from build123d import *

# Parameters (mm, degrees)
SKETCH1_W           = 107.95
SKETCH1_H           = 44.45
BOSS_EXTRUDE1_DEPTH = 69.85
SKETCH2_W           = 18.973953495
SKETCH2_H           = 6.048241647
CUT_EXTRUDE1_DEPTH  = 141.986
SKETCH3_W           = 38.080163228
SKETCH3_H           = 3.050825249
SKETCH3_W_2         = 51.430009823
CUT_EXTRUDE3_DEPTH  = 141.986
CUT_EXTRUDE4_DEPTH  = 141.986
SKETCH8_R           = 114.3
CUT_EXTRUDE6_DEPTH  = 33.274
SKETCH12_R          = 119.126
CUT_EXTRUDE7_DEPTH  = 7.874
SKETCH13_R          = 6.35
CUT_EXTRUDE8_DEPTH  = 20.574
SKETCH14_R          = 76.2
CUT_EXTRUDE9_DEPTH  = 7.874
SKETCH15_R          = 6.35
CUT_EXTRUDE10_DEPTH = 20.574
SKETCH16_R          = 4.826
CUT_EXTRUDE11_DEPTH = 81.28


with BuildPart() as part:
    # Sketch1 → Boss-Extrude1 (new body)
    with BuildSketch(Plane(origin=(0, 0, 0), x_dir=(1, 0, 0), z_dir=(0, 1, 0))):
        with Locations((2.544990177, 0.698624754)):
            Rectangle(SKETCH1_W, SKETCH1_H)
    extrude(amount=BOSS_EXTRUDE1_DEPTH)

    # Sketch2 → Cut-Extrude1 (cut)
    with BuildSketch(Plane(origin=(56.519990177, 0, 0), x_dir=(0, 0, -1), z_dir=(1, 0, 0))):
        with Locations((0.660601501, 3.024120824)):
            Rectangle(SKETCH2_W, SKETCH2_H)
    extrude(amount=-CUT_EXTRUDE1_DEPTH, mode=Mode.SUBTRACT)

    # Sketch3 → Cut-Extrude3 (cut)
    with BuildSketch(Plane.XY.offset(21.526375246)):
        with Locations((37.479908563, 1.525412625)):
            Rectangle(SKETCH3_W, SKETCH3_H)
        with Locations((-25.715004912, 1.525412625)):
            Rectangle(SKETCH3_W_2, SKETCH3_H)
    extrude(amount=-CUT_EXTRUDE3_DEPTH, mode=Mode.SUBTRACT)

    # Sketch7 → Cut-Extrude4 (cut)
    with BuildSketch(Plane.XY.offset(21.526375246)):
        Polygon((-51.430009823, 54.102), (-42.337897784, 69.85), (-51.430009823, 69.85), align=None)
    extrude(amount=-CUT_EXTRUDE4_DEPTH, mode=Mode.SUBTRACT)

    # Sketch8 → Cut-Extrude6 (cut)
    with BuildSketch(Plane(origin=(0, 69.85, 0), x_dir=(1, 0, 0), z_dir=(0, 1, 0))):
        with Locations((112.145990177, 0.825624754)):
            Circle(SKETCH8_R)
    extrude(amount=-CUT_EXTRUDE6_DEPTH, mode=Mode.SUBTRACT)

    # Sketch12 → Cut-Extrude7 (cut)
    with BuildSketch(Plane(origin=(0, 36.576, 0), x_dir=(1, 0, 0), z_dir=(0, 1, 0))):
        with Locations((112.145990177, 0.825624754)):
            Circle(SKETCH12_R)
    extrude(amount=CUT_EXTRUDE7_DEPTH, mode=Mode.SUBTRACT)

    # Sketch13 → Cut-Extrude8 (cut)
    with BuildSketch(Plane(origin=(0, 36.576, 0), x_dir=(1, 0, 0), z_dir=(0, 1, 0))):
        with Locations(Location((37.469990177, 0.825624754, 0), (0, 0, 270))):
            Circle(SKETCH13_R)
    extrude(amount=-CUT_EXTRUDE8_DEPTH, mode=Mode.SUBTRACT)

    # Sketch14 → Cut-Extrude9 (cut)
    with BuildSketch(Plane(origin=(0, 36.576, 0), x_dir=(1, 0, 0), z_dir=(0, 1, 0))):
        with Locations((107.319990177, 0.825624754)):
            Circle(SKETCH14_R)
    extrude(amount=-CUT_EXTRUDE9_DEPTH, mode=Mode.SUBTRACT)

    # Sketch15 → Cut-Extrude10 (cut)
    with BuildSketch(Plane(origin=(0, 69.85, 0), x_dir=(1, 0, 0), z_dir=(0, 1, 0))):
        with Locations(Location((-26.030009823, 0.825624754, 0), (0, 0, 270))):
            Circle(SKETCH15_R)
    extrude(amount=-CUT_EXTRUDE10_DEPTH, mode=Mode.SUBTRACT)

    # Sketch16 → Cut-Extrude11 (cut)
    with BuildSketch(Plane(origin=(0, 69.85, 0), x_dir=(1, 0, 0), z_dir=(0, 1, 0))):
        with Locations(Location((-26.030009823, 0.825624754, 0), (0, 0, 270))):
            Circle(SKETCH16_R)
        with Locations(Location((37.469990177, 0.825624754, 0), (0, 0, 270))):
            Circle(SKETCH16_R)
    extrude(amount=-CUT_EXTRUDE11_DEPTH, mode=Mode.SUBTRACT)


solid = part.part
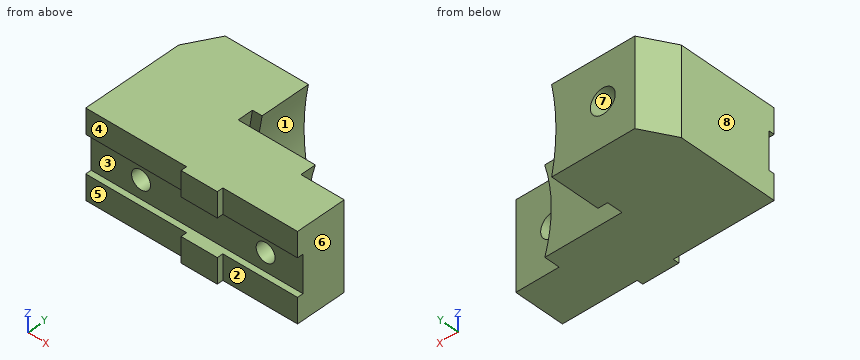
Geometry check sheet. Reference: the model listing, model coordinates, mm. Face numbers are marked on the shaded views. A direction names the side the tool comes from. Give positions to 0.01 mm unless a question says otherwise; leave off trailing zeros. Order: outer loops, then holes, each group sorted by start corner. A loop starts at its lowest first (then second) coordinate and runs counter-clockwise, first axis right, second up. Notation, with made-up numbers: M 11,37 L 35,37 A25 cw 35,61 Z; hole C 49.5,83.25 d1. An arc over 180 degrees is marked long. Use a Markdown table: item, result.
Item 1: Tool access check on the marked faces 1, 2, 3 and 4. Record the directions out of +Z, -Z, +X, -X, +Y, -Y that give a thin tool (end or side, any length) a straight path to the whole face; none if there is none.
Answers follow:
| item | result |
|---|---|
| face 1 | +X, +Y |
| face 2 | +Z, -Z, +X, -Y |
| face 3 | +X, -X, -Y |
| face 4 | +Z, -Z, -X, -Y |
Item 2: Section check B-B (z = -2). Record the cut outline in (x, y), and give its area (3 significant figures).
Answers follow:
| item | result |
|---|---|
| outline | M -51.43,6.05 L -30.71,6.05 L -30.71,49.28 L -32.27,49.28 L -32.27,69.85 L -42.34,69.85 L -51.43,54.1 Z; M -21.35,6.05 L 32.79,6.05 L 32.79,16 L 31.23,16 L 31.23,28.7 L 31.13,28.7 L 31.13,36.58 L -6.97,36.58 L -6.97,44.45 L -2.15,44.45 L -2.15,69.85 L -19.79,69.85 L -19.79,49.28 L -21.35,49.28 Z; M 42.15,6.05 L 56.52,6.05 L 56.52,28.7 L 43.71,28.7 L 43.71,16 L 42.15,16 Z |
| area | 3,710 mm2 |
Item 3: Material ranges on line 1 along X through (y, z) = (20.5, 1); line 2 along Y through (x, z) = (-5.5, 9.5); line 3 along Y through (x, z) = (13, 3), recorded low to high.
Answers follow:
| item | result |
|---|---|
| line 1 | x = -51.43 to -30.5, -21.56 to 31.39, 43.55 to 56.52 |
| line 2 | y = 3.05 to 36.58, 44.45 to 69.85 |
| line 3 | y = 6.05 to 36.58 |
Item 4: Depth check by flat-ended pin: P1, Ø1.5, axis at y = 1, z = 16.5, coming from the +X side; P2, Ø14, axis at x = -25.5, z = -14, coming from the -Y side; P3, Ø12.5, axis at x = 20, z = 6, coming from the +Y side. Enter the tip coordinate at first touch or a pass-through.
Answers follow:
| item | result |
|---|---|
| P1 | stops at x = 18.44 |
| P2 | stops at y = 3.05 |
| P3 | stops at y = 36.58 |
Item 5: Draft check along X on the marked faces 5, 6, 7 and 8. Enter one of: +X half, -X half, draft (parallel to the pull), parting line (faces both ways), or undercut.
Answers follow:
| item | result |
|---|---|
| face 5 | draft |
| face 6 | +X half |
| face 7 | undercut |
| face 8 | -X half |
Item 6: Section check A-A (y = 20). Record the cut outline in (x, z), and give its area (3 significant figures).
Answers follow:
| item | result |
|---|---|
| outline | M -51.43,-22.92 L 56.52,-22.92 L 56.52,21.53 L -51.43,21.53 Z; hole C -26.03,-0.83 d9.65; hole C 37.47,-0.83 d12.7 |
| area | 4,600 mm2 |
Item 7: Section check C-C (x = -37.5). Record the cut outline in (y, z), and give its area (3 significant figures).
Answers follow:
| item | result |
|---|---|
| outline | M 3.05,-22.92 L 69.85,-22.92 L 69.85,21.53 L 3.05,21.53 L 3.05,8.83 L 6.05,8.83 L 6.05,-10.15 L 3.05,-10.15 Z |
| area | 2,910 mm2 |
Item 8: Section check D-D (y = 58). Record the cut outline in (x, z).
Answers follow:
| item | result |
|---|---|
| outline | M -49.18,-22.92 L 0,-22.92 A114.3 cw 0.05,21.53 L -49.18,21.53 Z; hole C -26.03,-0.83 d12.7 |
